Source: CAD feature listing. Evaluate the final solid. Frame: model axes, mm. A direction names the side the tool comes from. Round coordinates to 2 decimals unless told otherwise and drop trailing zeros. Write each loop counter-clockwise with the first axis right and the second up, starting at its lowest first coordinate (ties: lowest second). Pieces come first, ordered by that corner, then holes.
Autodesk Inventor part; units mm, degrees
ref_plane "YZ Plane" through (0, 0, 0) normal (1, 0, 0) x (0, 1, 0)
ref_plane "XZ Plane" through (0, 0, 0) normal (0, 1, 0) x (-1, 0, 0)
ref_plane "XY Plane" through (0, 0, 0) normal (0, 0, 1) x (1, 0, 0)
sketch "Sketch1" plane through (0, 0, 0) normal (0, 0, 1) x (1, 0, 0)
  line L0 (0, 0) -> (36, 0)
  line L1 (36, 0) -> (36, 50)
  line L2 (36, 50) -> (0, 50)
  line L3 (0, 50) -> (0, 0)
  dimension "d0" = 36
  dimension "d1" = 50
extrude "Extrusion1" add sketch "Sketch1" along normal mid plane 36
sketch "Sketch2" plane through (0, 50, 18) normal (0, 1, 0) x (1, 0, 0)
  line L0 (28.15, 7.85) -> (7.85, 7.85)
  line L1 (7.85, 7.85) -> (7.85, 28.15)
  line L2 (7.85, 28.15) -> (28.15, 28.15)
  line L3 (28.15, 28.15) -> (28.15, 7.85)
  line L4 (28.15, 7.85) -> (7.85, 28.15) construction
  line L5 (7.85, 7.85) -> (28.15, 28.15) construction
  line L6 (0, 36) -> (0, 0)
  point P0 (0, 18)
  point P1 (18, 18)
  point P2 (0, 18)
  dimension "d4" = 18
  dimension "d5" = 20.3
  dimension "d6" = 20.3
extrude "Extrusion2" cut sketch "Sketch2" against normal blind 33
sketch "Sketch3" plane through (0, 0, 18) normal (0, 0, 1) x (1, 0, 0)
  line L0 (0, 50) -> (0, 0)
  line L1 (0, 0) -> (36, 0)
  point P0 (18, 12)
  dimension "d9" = 18
  dimension "d10" = 12
hole "Hole1" at (18, 12, 18) direction (0, 0, -1) diameter 6.2 end through all
sketch "Sketch8" plane through (7.85, 50, -10.15) normal (0, 0, 1) x (1, 0, 0)
  point P0 (-7.85, -50)
sketch "Sketch11" plane through (0, 0, 18) normal (-1, 0, 0) x (0, 0, 1)
  circle A0 centre (-18, 24) radius 3.1
  line L0 (0, 50) -> (0, 0)
  line L1 (-7.85, 17) -> (-28.15, 17)
  point P0 (-18, 0)
  dimension "d41" = 6.2
  dimension "d42" = 18
  dimension "d43" = 7
extrude "Extrusion6" cut sketch "Sketch11" against normal through all
fillet "Fillet1" radius 10 4 edges at (36, 25, 18) (0, 25, 18) (0, 25, -18) (36, 25, -18)
fillet "Fillet2" radius 5 8 edges at (18, 0, 18) (33.0711, 0, 15.0711) (36, 0, 0) (33.0711, 0, -15.0711) (18, 0, -18) (2.9289, 0, -15.0711) (0, 0, 0) (2.9289, 0, 15.0711)
fillet "Fillet3" radius 6.8 8 edges at (33.0711, 50, 15.0711) (18, 50, 18) (2.9289, 50, 15.0711) (0, 50, 0) (2.9289, 50, -15.0711) (18, 50, -18) (33.0711, 50, -15.0711) (36, 50, 0)
properties part number "arm_collar"
1) Section query D-D on x = 18. Return the cut outline in (y, z).
Taken from the geometry:
outline: (0, -13) arc R5 ccw to (5, -18) - (8.9, -18) - (8.9, 18) - (5, 18) arc R5 ccw to (0, 13) - close; (15.1, -18) - (43.2, -18) arc R6.8 ccw to (50, -11.2) - (50, -10.15) - (17, -10.15) - (17, 10.15) - (50, 10.15) - (50, 11.2) arc R6.8 ccw to (43.2, 18) - (15.1, 18) - close
2) Pull-direction query (Z, two-part tool) for faces 1 (the face through (18, 34, -10.15)), 2 (the face through (19.886, 14.46, -0.252)), 3 (the face through (18.112, 48.061, 15.955)); classes: released by +Z, released by -Z, zero draft, split by the parting line, or undercut.
Taken from the geometry:
face 1: undercut
face 2: zero draft
face 3: released by +Z
3) Section query B-B on y = 12. Return the cut outline in (x, z).
Taken from the geometry:
outline: (0, -8) arc R10 ccw to (10, -18) - (14.9, -18) - (14.9, 18) - (10, 18) arc R10 ccw to (0, 8) - close; (21.1, -18) - (26, -18) arc R10 ccw to (36, -8) - (36, 8) arc R10 ccw to (26, 18) - (21.1, 18) - close
4) Section query A-A on z = 0. Return the cut outline in (x, y), then the cut area to 3 significant figures.
Taken from the geometry:
outline: (0, 5) arc R5 ccw to (5, 0) - (31, 0) arc R5 ccw to (36, 5) - (36, 20.9) - (28.15, 20.9) - (28.15, 17) - (7.85, 17) - (7.85, 20.9) - (0, 20.9) - close; (0, 27.1) - (7.85, 27.1) - (7.85, 50) - (6.8, 50) arc R6.8 ccw to (0, 43.2) - close; (28.15, 27.1) - (36, 27.1) - (36, 43.2) arc R6.8 ccw to (29.2, 50) - (28.15, 50) - close; hole circle Ø6.2 at (18, 12)
area: 972 mm2
5) Contact query for flat-ended pins moving along their axis: P1, Ø1, axis at y = 15, z = -12.5, coming from the -X side; P2, Ø5, axis at y = 18, z = 13.5, coming from the -X side; P3, Ø10, axis at x = 13.5, z = 0, coming from the +Y side. Output: stop coordinate, or through.
Taken from the geometry:
P1: stops at x = 0.83
P2: stops at x = 0.46
P3: stops at y = 17
6) Reachability of faces 4 (the face through (35, 2, 0)), 5 (the face through (18, 17, 0)) from +Z, -Z, +X, -X, +Y, -Y: full face, straight path, thin tool, end or side. Return the list, or none.
Taken from the geometry:
face 4: +Z, -Z, +X, -Y
face 5: +Y
7) Section query C-C on y = 34.5. Return the cut outline in (x, z).
Taken from the geometry:
outline: (0, -8) arc R10 ccw to (10, -18) - (26, -18) arc R10 ccw to (36, -8) - (36, 8) arc R10 ccw to (26, 18) - (10, 18) arc R10 ccw to (0, 8) - close; hole (7.85, -10.15) - (28.15, -10.15) - (28.15, 10.15) - (7.85, 10.15) - close
8) Material intervals for line 1 (X direction, y = 41.5, z = -2); line 2 (Z direction, x = 20, y = 39.5); line 3 (Y direction, x = 18, z = 5), sorted ascending.
Taken from the geometry:
line 1: x = 0 to 7.85, 28.15 to 36
line 2: z = -18 to -10.15, 10.15 to 18
line 3: y = 0 to 8.9, 15.1 to 17
